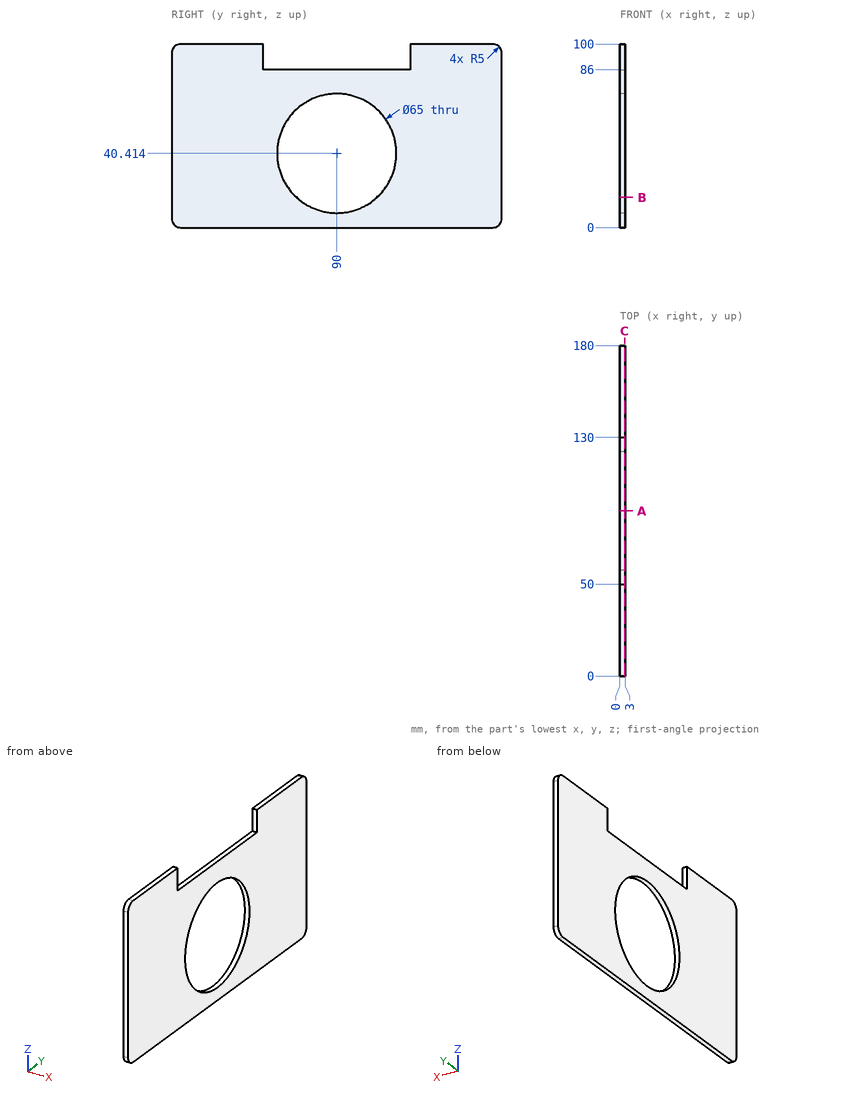
Source: three-view drawing plus pictorial views. Frame: mm from the lowest corner of the part. Give positions to 0.01 mm unless a question says otherwise; leave off trailing zeros. Write each loop counter-clockwise with the first axis right and the second up, starting at its lowest first coordinate (ties: lowest second). Pieces come first, ordered by that corner, then holes.
(1) Cut plane A-A, the plane y = 90. Return loops of the section in (x, z), then the cut area to 3 significant figures.
(2) First-contact query: P1, Ø6, axis at y = 110.5, z = 81, coming from the -X side. Flat tip, straight axial feed; report the tip coordinate or a pass-through.
(3) Cut plane B-B, the plane z = 16.5. Return loops of the section in (x, y), then the cut area to 3 significant figures.
(4) Cut plane C-C, the plane x = 2.55. Return loops of the section in (y, z), then the cut area to 3 significant figures.
(5) Ray query, line 1 (Z direction, x = 1.75, y = 90); line 2 (Y direction, x = 0.8, z = 27); line 3 (Y direction, x = 1.3, z = 24.5). Return the intervals inside material, ascending.
Values follow:
1. outline: (0, 0) - (3, 0) - (3, 7.91) - (0, 7.91) - close; (0, 72.91) - (3, 72.91) - (3, 86) - (0, 86) - close
1. area: 63.0 mm2
2. P1: stops at x = 0
3. outline: (0, 0) - (3, 0) - (3, 67.99) - (0, 67.99) - close; (0, 112.01) - (3, 112.01) - (3, 180) - (0, 180) - close
3. area: 408 mm2
4. outline: (0, 5) arc R5 ccw to (5, 0) - (175, 0) arc R5 ccw to (180, 5) - (180, 95) arc R5 ccw to (175, 100) - (130, 100) - (130, 86) - (50, 86) - (50, 100) - (5, 100) arc R5 ccw to (0, 95) - close; hole circle Ø65 at (90, 40.41)
4. area: 13,500 mm2
5. line 1: z = 0 to 7.91, 72.91 to 86
5. line 2: y = 0 to 60.4, 119.6 to 180
5. line 3: y = 0 to 61.66, 118.34 to 180
